Design review of the part built by this model. Coordinates are the model's own, in mm. A direction names the side the tool comes from. Coordinates: 2 decimals unless noted, no trailing zeros. Write each loop counter-clockwise with the first axis right and the second up, starting at its lowest first coordinate (ties: lowest second). Pieces come first, ordered by that corner, then holes. Notation, with made-up numbers: (86.25, 63) - (121.25, 63) arc R34 cw to (121.25, 95) - close; hole circle Ø10 at (15.5, 85.5). An arc over 180 degrees is marked (long way). Answer as a JSON object with one key per item and string values.
```python
from build123d import *

# Parameters (mm, degrees)
BOSS_EXTRUDE1_DEPTH = 3.175
FILLET1_R           = 3.175


with BuildPart() as part:
    # Sketch1 → Boss-Extrude1 (new body)
    with BuildSketch(Plane.XY):
        Polygon((0, 5.842), (6.35, 5.842), (6.35, 0), (12.7, 0), (12.7, 5.842), (19.05, 5.842), (19.05, 9.017), (3.175, 12.192), (-9.525, 9.017), (-9.525, 5.842), (-6.35, 5.842), (-6.35, 0), (0, 0), align=None)
    extrude(amount=BOSS_EXTRUDE1_DEPTH)

    # Fillet1
    fillet1_edges = [part.edges().sort_by_distance(p)[0] for p in [
        (-9.525, 9.017, 1.5875),
        (3.175, 12.192, 1.5875),
        (19.05, 9.017, 1.5875),
    ]]
    fillet(fillet1_edges, radius=FILLET1_R)


solid = part.part
```
(1) The part is to be moulded in two halves that separate along X. For faces 1 (the face through (-8.83, 8.52, 1.61)), 2 (the face through (0, 3, 2)), 3 (the face through (-8, 5.842, 2)), say which applies: pulls with the +X half, pulls with the -X half, needs draft (parallel to the pull), parting line crosses it, or undercut.
Solved:
{"face 1": "pulls with the -X half", "face 2": "undercut", "face 3": "needs draft"}
(2) For pin 1 (1 mm diameter, centred on x = -7.5, z = 1, fed in from -Y); pin 2 (1 mm diameter, centred on y = 2.5, z = 2, fed in from -X), all flat-tipped, find the tip position at first contact; note any pin that passes through.
Solved:
{"pin 1": "stops at y = 5.84", "pin 2": "stops at x = -6.35"}
(3) Take a section at A-A, the plane y = 3.25. Write out the cut boundary in (x, z) (3 decimals).
Solved:
{"outline": "(-6.35, 0) - (0, 0) - (0, 3.175) - (-6.35, 3.175) - close; (6.35, 0) - (12.7, 0) - (12.7, 3.175) - (6.35, 3.175) - close"}
(4) Tool access review of faces 4 (the face through (-6.35, 3, 2)), 5 (the face through (16, 5.842, 2)), 6 (the face through (6.35, 3, 2)): name each direction out of +Z, -Z, +X, -X, +Y, -Y from which nothing blocks a thin tool from reaching the whole face with its end or side.
Solved:
{"face 4": "+Z, -Z, -X, -Y", "face 5": "+Z, -Z, +X, -Y", "face 6": "+Z, -Z, -Y"}
(5) Take a section at D-D, the plane y = 10.75. Write out the cut boundary in (x, z) (3 decimals), and give its area (3 significant figures).
Solved:
{"outline": "(-2.593, 0) - (10.385, 0) - (10.385, 3.175) - (-2.593, 3.175) - close", "area": "41.2 mm^2"}
(6) To check wall thickness, follow line 1 (X direction, y = 2.5, z = 2.15); line 2 (Y direction, x = 3.25, z = 1.1); line 3 (X direction, y = 6.5, z = 1.6) (3 decimals). State the ranges of each line that lie inside material, in increasing order. Write a range as from..to.
Solved:
{"line 1": "x = -6.35..0, 6.35..12.7", "line 2": "y = 5.84..12.11", "line 3": "x = -9.525..19.049"}
(7) Take a section at B-B, the plane z = 2.9. Write out the cut boundary in (x, y) (3 decimals), and give its area (3 significant figures).
Solved:
{"outline": "(-9.525, 5.842) - (-6.35, 5.842) - (-6.35, 0) - (0, 0) - (0, 5.842) - (6.35, 5.842) - (6.35, 0) - (12.7, 0) - (12.7, 5.842) - (19.05, 5.842) - (19.05, 6.414) arc R3.175 ccw to (16.498, 9.527) - (3.875, 12.052) arc R3.175 ccw to (2.482, 12.019) - (-7.12, 9.618) arc R3.175 ccw to (-9.525, 6.538) - close", "area": "208 mm^2"}
(8) Take a section at C-C, the plane x = 14.75. Write out the cut boundary in (y, z) (3 decimals), and give its area (3 significant figures).
Solved:
{"outline": "(5.842, 0) - (9.877, 0) - (9.877, 3.175) - (5.842, 3.175) - close", "area": "12.8 mm^2"}
